Geometry check sheet. Reference: the model listing, model coordinates, mm. A direction names the side the tool comes from. Round coordinates to 2 decimals unless told otherwise and drop trailing zeros. Loops run counter-clockwise (first coordinate to the right, second up) from the corner with the lowest first, then second, coordinate; pieces in that order, holes last. Notation, with made-up numbers: (-16, -10.5) -> (19, -10.5) arc R21 ccw to (19, -6.5) -> close; hole circle Ø6 at (1, 56.25). An arc over 180 degrees is marked (long way). Use a Markdown table: item, result. Add a question column.
Q1. Sectioned sample at A-A, the plane x = -54. Enter the section's corners in (y, z).
Q2. Set-up check for faces 1 (the face through (-39, 10, -58.42)), 2 (the face through (-7.397, 80.204, -58.702)): record each of +Z, -Z, +X, -X, +Y, -Y from which the full face is reachable in a straight line by a thin tool's end or side.
Q3. Sectioned sample at C-C, the plane y = 95.5. Enter the section's corners in (x, z).
Q4. Material ranges on L1, parallel to Y at x = -47.5, z = 22.5; L2, parallel to Z at x = -49, y = 0.5; L3, parallel to X at y = 86, z = 10, recorded low to high.
Q5. Sectioned sample at B-B, the plane z = -45. Enter the section's corners in (x, y).
Q6. Gauge pin test, flat ends, axial feed: P1, Ø10, axis at x = -79.5, z = -74.5, coming from the +Y side; P2, Ø6, axis at x = -15.5, y = 19, coming from the -Z side; P3, Ø1.5, axis at x = -77, y = 5, coming from the -Z side; P4, Ø6, axis at y = -13, z = 42.5, coming from the -X side. Record the tip position at first contact, or that the pin passes through.
Q7. Sectioned sample at D-D, the plane x = -13.5. Enter the section's corners in (y, z).
Q8. Release check for a two-part mould opening along Y. For faces 3 (the face through (25.4, 91, 1)), 4 (the face through (-50.745, 123.176, -1.679)), 5 (the face through (-56.3, 15.6, -0.8)) record: released by +Y, released by -Y, zero draft, split by the parting line, or undercut.
```python
from build123d import *

# Parameters (mm, degrees)
BOSS_EXTRUDE2_DEPTH      = 25.4
BOSS_EXTRUDE2_DEPTH_BACK = 97.79
CUT_EXTRUDE1_DEPTH       = 251.97847836
CUT_EXTRUDE2_DEPTH       = 58.42
CUT_EXTRUDE2_DEPTH_BACK  = 58.42
SKETCH4_R                = 58.42


with BuildPart() as part:
    # Sketch1 → Revolve1 (revolve)
    with BuildSketch(Plane.XY):
        with BuildLine():
            Line((-195.58, 25.4), (0, 25.4))
            ThreePointArc((0, 25.4), (-97.79, 123.19), (-195.58, 25.4))
        make_face()
    revolve(axis=Axis((-195.58, 25.4, 0), (1, 0, 0)))

    # Sketch2 → Boss-Extrude2 (add, two sides: drawn at the far end of the back side and taken through both)
    with BuildSketch(Plane(origin=(0, 0, 0), x_dir=(0, 0, -1), z_dir=(1, 0, 0)).offset(-BOSS_EXTRUDE2_DEPTH_BACK)):
        with BuildLine():
            Line((-92.046530081, 58.42), (92.046530081, 58.42))
            ThreePointArc((92.046530081, 58.42), (0, 123.19), (-92.046530081, 58.42))
        make_face()
    extrude(amount=BOSS_EXTRUDE2_DEPTH + BOSS_EXTRUDE2_DEPTH_BACK)

    # Sketch3 → Cut-Extrude1 (cut, through all)
    with BuildSketch(Plane(origin=(0, 0, 0), x_dir=(1, 0, 0), z_dir=(0, 1, 0))):
        Polygon((25.4, -38.1), (25.4, 38.1), (-97.79, 115.482462919), (50.8, 115.482462919), (50.8, -115.482462919), (-97.79, -115.482462919), align=None)
    extrude(amount=CUT_EXTRUDE1_DEPTH, mode=Mode.SUBTRACT)

    # Sketch4 → Cut-Extrude2 (cut, two sides: drawn at the far end of the back side and taken through both)
    with BuildSketch(Plane.XY.offset(-CUT_EXTRUDE2_DEPTH_BACK)):
        Circle(SKETCH4_R)
    extrude(amount=CUT_EXTRUDE2_DEPTH + CUT_EXTRUDE2_DEPTH_BACK, mode=Mode.SUBTRACT)


solid = part.part
```
Values:
| question | item | result |
|---|---|---|
| 1 | outline | (58.42, -87.98) -> (68.1, -87.98) arc R97.79 ccw to (68.1, 87.98) -> (58.42, 87.98) -> (58.42, 80.96) arc R87.44 ccw (long way) to (58.42, -80.96) -> close; hole (-22.29, -58.42) -> (22.29, -58.42) -> (22.29, 58.42) -> (-22.29, 58.42) -> close |
| 2 | face 1 | +X |
| 2 | face 2 | -Z, +X, +Y, -Y |
| 3 | outline | (-97.79, -68.18) -> (-22.49, -68.18) -> (25.4, -38.1) -> (25.4, 38.1) -> (-22.49, 68.18) -> (-97.79, 68.18) arc R68.18 ccw to start |
| 4 | L1 | -55.39 to -34.01, 34.01 to 120.57 |
| 4 | L2 | -81.01 to -58.42, 58.42 to 81.01 |
| 4 | L3 | -173.89 to 25.4 |
| 5 | outline | (-97.79, 112.22) arc R86.82 ccw (long way) to (-41.72, -40.89) arc R58.42 cw to (-16.55, 56.03) arc R86.82 ccw to (-17.49, 58.42) -> (14.42, 58.42) -> (14.42, 112.22) -> close |
| 6 | P1 | y = 94.19 |
| 6 | P2 | through |
| 6 | P3 | z = -93.58 |
| 6 | P4 | x = -179.13 |
| 7 | outline | (56.84, -38.34) arc R49.58 ccw to (58.42, -36.98) -> (58.42, -62.54) -> (100.58, -62.54) arc R97.79 ccw to (100.58, 62.54) -> (58.42, 62.54) -> (58.42, 36.98) arc R49.58 ccw to (56.84, 38.34) -> close |
| 8 | face 3 | zero draft |
| 8 | face 4 | released by +Y |
| 8 | face 5 | undercut |
